CAD build for the part. Positions are in the model's coordinates, mm. A direction names the side the tool comes from. Coordinates: 2 decimals unless noted, no trailing zeros. Loops run counter-clockwise (first coordinate to the right, second up) from the corner with the lowest first, then second, coordinate; pieces in that order, holes last.
1) Saw through at B-B, the plane x = 1.25. Write the cut outline in (y, z).
2) Wall check: line 1 along Y through (x, z) = (1, 5.05); line 2 along Z through (x, y) = (-0.25, -32.55); line 3 along Z through (x, y) = (-12.5, -33.1). Give the ranges that are in metal, low to high.
3) Saw through at A-A, the plane z = 7. Write the cut outline in (x, y), and give its area (3 significant figures).
4) Which spindle directions (+Z, -Z, +X, -X, +Y, -Y) get a long thin tool onto all of the face, cutting with end or side? Do faces 1 (the cylindrical face through (-12.2, -32.6, 7)), 2 (the cylindrical face through (3.2, -32.6, 7)), 3 (the flat face through (-4.6, -32.6, 5.8)). Say none if no direction does.
5) Saw through at D-D, the plane z = 5.2. Write the cut outline in (x, y), and give its area (3 significant figures).
6) Pin check, flat tip, straight feed: pin 1 Ø1.5 at (x, y) = (-1.5, -31.5) entering from +Z. Stop position of the tip, or through.
7) Saw through at C-C, the plane y = -32.4. Write the cut outline in (x, z).
```python
from build123d import *

# Parameters (mm, degrees)
EXTRUDE010_DEPTH = 1
EXTRUDE009_DEPTH = 2.4
CHAMFER005_SIZE2 = 1.5
CHAMFER005_SIZE  = 0.8


with BuildPart() as extrude010:
    # Sketch011 (on Sketch) → Extrude010 (new body)
    with BuildSketch(Plane.XZ.offset(33)):
        with BuildLine():
            ThreePointArc((-11, 10), (-14, 7), (-11, 4))
            Line((-11, 4), (2, 4))
            ThreePointArc((2, 4), (5, 7), (2, 10))
            Line((2, 10), (-11, 10))
        make_face()
    extrude(amount=EXTRUDE010_DEPTH)


with BuildPart() as obj1:
    # Sketch010 (on Sketch) → Extrude009 (new body)
    with BuildSketch(Plane.XZ.offset(33)):
        with BuildLine():
            ThreePointArc((-11, 8.2), (-12.2, 7), (-11, 5.8))
            Line((-11, 5.8), (2, 5.8))
            ThreePointArc((2, 5.8), (3.2, 7), (2, 8.2))
            Line((2, 8.2), (-11, 8.2))
        make_face()
    extrude(amount=-EXTRUDE009_DEPTH)

    # Connect002: union Extrude010
    add(extrude010.part)

    # Chamfer005
    chamfer005_edges = [obj1.edges().sort_by_distance(p)[0] for p in [
        (-4.5, -30.6, 8.2),
    ]]
    chamfer005_side = obj1.faces().sort_by_distance((-4.5, -30.6, 7))[0]
    chamfer(chamfer005_edges, length=CHAMFER005_SIZE, length2=CHAMFER005_SIZE2, reference=chamfer005_side)


solid = obj1.part
```
Data:
1. outline: (-34, 4) - (-33, 4) - (-33, 5.8) - (-32.1, 5.8) - (-30.6, 6.6) - (-30.6, 7.4) - (-32.1, 8.2) - (-33, 8.2) - (-33, 10) - (-34, 10) - close
2. line 1: y = -34 to -33
2. line 2: z = 5.8 to 8.2
2. line 3: z = 4.4 to 9.6
3. outline: (-14, -34) - (5, -34) - (5, -33) - (3.2, -33) - (3.2, -32.1) - (2.4, -30.6) - (-11.4, -30.6) - (-12.2, -32.1) - (-12.2, -33) - (-14, -33) - close
3. area: 54.8 mm2
4. face 1: -X, +Y
4. face 2: +X, +Y
4. face 3: -Z, +X, -X, +Y
5. outline: (-13.4, -34) - (4.4, -34) - (4.4, -33) - (-13.4, -33) - close
5. area: 17.8 mm2
6. pin 1: stops at z = 8.2
7. outline: (-11, 5.8) - (2, 5.8) arc R1.2 ccw to (2, 8.2) - (-11, 8.2) arc R1.2 ccw to start
